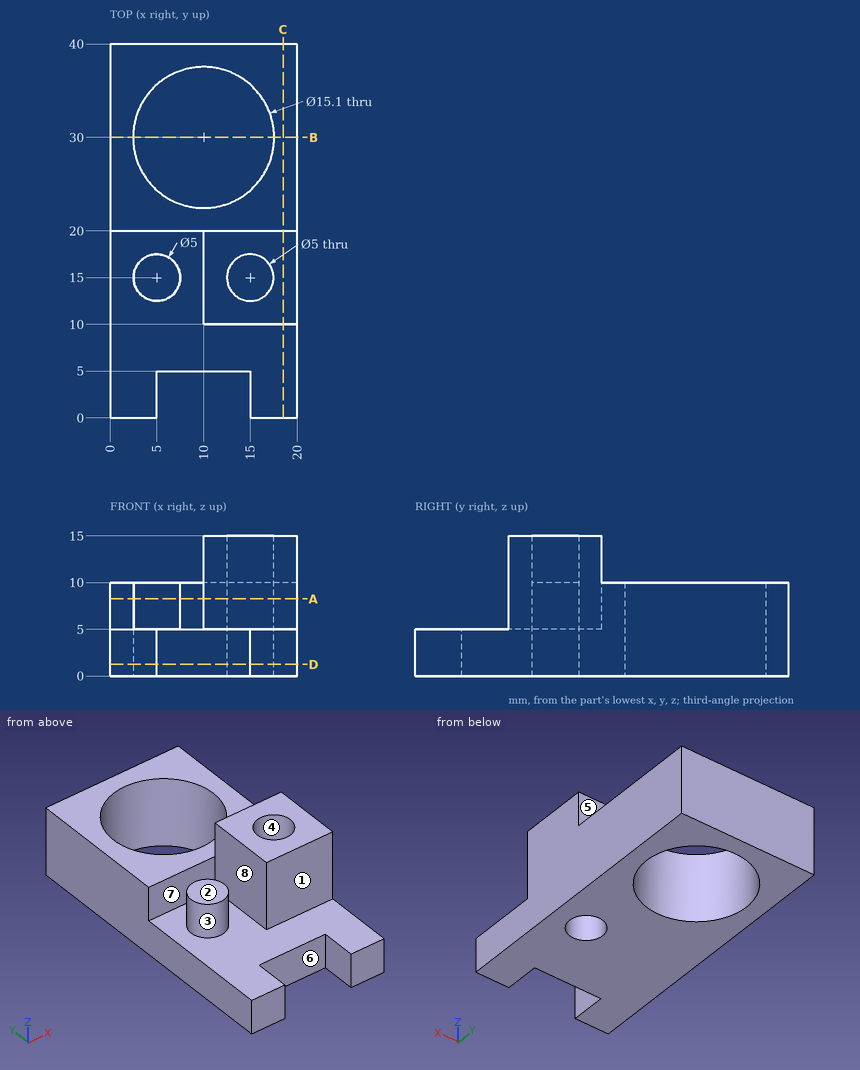
Source: three-view drawing plus pictorial views. Frame: mm from the lowest corner of the part. A direction names the side the tool comes from. Round coordinates to 2 decimals unless told otherwise and drop trailing zeros. Loops run counter-clockwise (first coordinate to the right, second up) from the corner with the lowest first, then second, coordinate; pieces in that order, holes last. Notation, with made-up numbers: M -36,15.25 L 8,15.25 A17 ccw 8,48.25 Z; hole C -6,62.5 d8. An arc over 180 degrees is marked long. Put each result on its own line as item: value.
(1) Pull-direction query (Y, two-part tool) for the marked faces 1, 2 and 3; classes: released by +Y, released by -Y, zero draft, split by the parting line, or undercut.
Solutions:
face 1: released by -Y
face 2: zero draft
face 3: undercut
(2) First-contact query: pin 1 (12 mm diameter, centred on x = 4.5, y = 5, fed in from +Z); pin 2 (10 mm diameter, centred on x = 14, y = 29, fed in from +Z); pin 3 (2.5 mm diameter, centred on x = 7.5, z = 8.5, fed in from -Y). Flat tips, straight axial feed; report the tip coordinate or a pass-through.
Solutions:
pin 1: z = 5
pin 2: z = 10
pin 3: y = 12.83
(3) Section B-B, the plane y = 30. Return loops of the section in (x, z).
Solutions:
outline: M 0,0 L 2.45,0 L 2.45,10 L 0,10 Z; M 17.55,0 L 20,0 L 20,10 L 17.55,10 Z
(4) Section A-A, the plane z = 8.25. Return loops of the section in (x, y).
Solutions:
outline: M 0,20 L 10,20 L 10,10 L 20,10 L 20,40 L 0,40 Z; C 5,15 d5; hole C 10,30 d15.1; hole C 15,15 d5
(5) Section C-C, the plane x = 18.5. Return loops of the section in (y, z), and give its area (3 significant figures).
Solutions:
outline: M 0,0 L 40,0 L 40,10 L 20,10 L 20,15 L 10,15 L 10,5 L 0,5 Z
area: 400 mm²
(6) Ray query, line 1 (Y direction, x = 15, z = 6.25); line 2 (X direction, y = 15.5, z = 6.5); line 3 (Y direction, x = 15, z = 11.25). Return the intervals inside material, ascending. Write a range as [from, to].
Solutions:
line 1: [10, 12.5], [17.5, 24.34], [35.66, 40]
line 2: [2.55, 7.45], [10, 12.55], [17.45, 20]
line 3: [10, 12.5], [17.5, 20]
(7) Access query for the marked faces 4, 5, 6, 7 and 8. Directions: +Z, -Z, +X, -X, +Y, -Y. A direction counts if a zero-diameter tool reaches every point of the face in a straight line with its end or side. Return the directions, or none.
Solutions:
face 4: +Z, -Z
face 5: +Z, +X, -X, +Y
face 6: +Z, -Z, -Y
face 7: +Z, -X
face 8: +Z, -Y
(8) Section D-D, the plane z = 1.25. Return loops of the section in (x, y), and give its area (3 significant figures).
Solutions:
outline: M 0,0 L 5,0 L 5,5 L 15,5 L 15,0 L 20,0 L 20,40 L 0,40 Z; hole C 10,30 d15.1; hole C 15,15 d5
area: 551 mm²
